Verification items for the finished model (mm, model axes). Face numbers are marked on the shaded views. A direction names the side the tool comes from. Give positions to 0.01 mm unless a question says otherwise; leave off trailing zeros. One line per question, with ' | ' between items. Start each with the question number.
Q1. Go/stop test with flat-tipped pins: pin 1 (2 mm diameter, centred on x = 43, y = -43.5, fed in from -Z); pin 2 (1 mm diameter, centred on x = 48, z = 2, fed in from -Y); pin 3 (4 mm diameter, centred on y = 26, z = 4.5, fed in from -X). Record where each tip stops, or that it passes through.
Q2. Mould release check, pull along X, two halves, no side actions. Record for the marked faces 3 and 4: released by +X, released by -X, zero draft, split by the parting line, or undercut.
Q3. Section check A-A on x = 26.5. Give the number of separate pieces and of enclosed holes in the cut face, plus the area to 3 significant figures.
Q4. Access from +Z, -Z, +X, -X, +Y, -Y to the whole of each face (thin tool, end or side, straight path). Record for the marked faces 1 and 2.
Q5. Material ranges on probe 1 along X at (y, z) = (22, 5.5); probe 2 along Y at (x, z) = (-28, 1.5); probe 3 along Y at (x, z) = (-18, 6.75), recorded low to high. Write a range as [from, to].
Autodesk Inventor part; units mm, degrees
ref_plane "Work Plane3" through (19.3185, -5.1764, 0) normal (-0.9659, 0.2588, 0) x (-0.2588, -0.9659, 0)
ref_plane "YZ Plane" through (0, 0, 0) normal (1, 0, 0) x (0, 1, 0)
ref_plane "XZ Plane" through (0, 0, 0) normal (0, 1, 0) x (-1, 0, 0)
sketch "Sketch1" plane through (0, 0, 0) normal (0, 0, 1) x (1, 0, 0)
  circle A0 centre (0, 0) radius 72.5
  circle A1 centre (0, 0) radius 67.5
  circle A2 centre (0, 0) radius 4
  line L0 (0, 20) -> (0, 60)
  arc A3 (0, 20) -> (-10, 17.3205) centre (0, 0) ccw
  line L1 (0, 0) -> (-10, 17.3205) construction
  line L2 (0, 0) -> (0, 20) construction
  arc A4 (0, 60) -> (-30, 51.9615) centre (0, 0) ccw
  line L3 (0, 0) -> (-30, 51.9615) construction
  line L4 (0, 0) -> (0, 60) construction
  line L5 (-10, 17.3205) -> (-30, 51.9615)
  line L6 (-17.3205, 10) -> (-51.9615, 30)
  arc A5 (-17.3205, 10) -> (-20, 0) centre (0, 0) ccw
  line L7 (0, 0) -> (-20, 0) construction
  line L8 (0, 0) -> (-17.3205, 10) construction
  arc A6 (-51.9615, 30) -> (-60, 0) centre (0, 0) ccw
  line L9 (0, 0) -> (-60, 0) construction
  line L10 (0, 0) -> (-51.9615, 30) construction
  line L11 (-20, 0) -> (-60, 0)
  line L12 (-17.3205, -10) -> (-51.9615, -30)
  arc A7 (-17.3205, -10) -> (-10, -17.3205) centre (0, 0) ccw
  line L13 (0, 0) -> (-10, -17.3205) construction
  line L14 (0, 0) -> (-17.3205, -10) construction
  arc A8 (-51.9615, -30) -> (-30, -51.9615) centre (0, 0) ccw
  line L15 (0, 0) -> (-30, -51.9615) construction
  line L16 (0, 0) -> (-51.9615, -30) construction
  line L17 (-10, -17.3205) -> (-30, -51.9615)
  line L18 (0, -20) -> (0, -60)
  arc A9 (0, -20) -> (10, -17.3205) centre (0, 0) ccw
  line L19 (0, 0) -> (10, -17.3205) construction
  line L20 (0, 0) -> (0, -20) construction
  arc A10 (0, -60) -> (30, -51.9615) centre (0, 0) ccw
  line L21 (0, 0) -> (30, -51.9615) construction
  line L22 (0, 0) -> (0, -60) construction
  line L23 (10, -17.3205) -> (30, -51.9615)
  line L24 (17.3205, -10) -> (51.9615, -30)
  arc A11 (17.3205, -10) -> (20, 0) centre (0, 0) ccw
  line L25 (0, 0) -> (20, 0) construction
  line L26 (0, 0) -> (17.3205, -10) construction
  arc A12 (51.9615, -30) -> (60, 0) centre (0, 0) ccw
  line L27 (0, 0) -> (60, 0) construction
  line L28 (0, 0) -> (51.9615, -30) construction
  line L29 (20, 0) -> (60, 0)
  line L30 (17.3205, 10) -> (51.9615, 30)
  arc A13 (17.3205, 10) -> (10, 17.3205) centre (0, 0) ccw
  line L31 (0, 0) -> (10, 17.3205) construction
  line L32 (0, 0) -> (17.3205, 10) construction
  arc A14 (51.9615, 30) -> (30, 51.9615) centre (0, 0) ccw
  line L33 (0, 0) -> (30, 51.9615) construction
  line L34 (0, 0) -> (51.9615, 30) construction
  line L35 (10, 17.3205) -> (30, 51.9615)
  point P0 (0, 10)
  point P1 (-2.5882, 9.6593)
  point P2 (-5, 8.6603)
  point P3 (-7.0711, 7.0711)
  point P4 (-8.6603, 5)
  point P5 (-9.6593, 2.5882)
  point P6 (-10, 0)
  point P7 (-9.6593, -2.5882)
  point P8 (-8.6603, -5)
  point P9 (-7.0711, -7.0711)
  point P10 (-5, -8.6603)
  point P11 (-2.5882, -9.6593)
  point P12 (0, -10)
  point P13 (2.5882, -9.6593)
  point P14 (5, -8.6603)
  point P15 (7.0711, -7.0711)
  point P16 (8.6603, -5)
  point P17 (9.6593, -2.5882)
  point P18 (10, 0)
  point P19 (9.6593, 2.5882)
  point P20 (8.6603, 5)
  point P21 (7.0711, 7.0711)
  point P22 (5, 8.6603)
  point P23 (2.5882, 9.6593)
  point P24 (15.5291, -57.9555)
  point P25 (30, -51.9615)
  point P26 (42.4264, -42.4264)
  point P27 (51.9615, -30)
  point P28 (57.9555, -15.5291)
  point P29 (60, 0)
  point P30 (57.9555, 15.5291)
  point P31 (51.9615, 30)
  point P32 (42.4264, 42.4264)
  point P33 (30, 51.9615)
  point P34 (15.5291, 57.9555)
  point P35 (0, 60)
  point P36 (-15.5291, 57.9555)
  point P37 (-30, 51.9615)
  point P38 (-42.4264, 42.4264)
  point P39 (-51.9615, 30)
  point P40 (-57.9555, 15.5291)
  point P41 (-60, 0)
  point P42 (-57.9555, -15.5291)
  point P43 (-51.9615, -30)
  point P44 (-42.4264, -42.4264)
  point P45 (-30, -51.9615)
  point P46 (-15.5291, -57.9555)
  dimension "d1" = 135
  dimension "d2" = 8
  dimension "d11" = 40
  dimension "d12" = 20
  dimension "d13" = 30
  dimension "d14" = 30
  dimension "d17" = 360
  dimension "d34" = 10
  dimension "d37" = 360
  dimension "d48" = 360
  dimension "d57" = 145
extrude "Extrusion1" add sketch "Sketch1" along normal blind 10 contours A1
extrude "Extrusion2" add sketch "Sketch1" along normal blind 5.5 contours A0
hole "Hole2" at (-2.5882, -9.6593, 0) at (-7.0711, 7.0711, 0) at (9.6593, 2.5882, 0) direction (0, 0, 1) diameter 4 end through all counterbore diameter 7 counterbore depth 4
hole "Hole3" at (42.4264, -42.4264, 0) at (-57.9555, -15.5291, 0) at (15.5291, 57.9555, 0) direction (0, 0, 1) diameter 4 end through all counterbore diameter 7 counterbore depth 4
chamfer "Chamfer2" distance 3.5 distance2 5 1 edges at (-72.5, 0, 5.5) measured on face at (72.06, -7.9756, 1.8333)
ref_plane "Work Plane3" through (19.3185, -5.1764, 0) normal (-0.9659, 0.2588, 0) x (-0.2588, -0.9659, 0)
sketch "Sketch3" plane through (19.3185, -5.1764, 0) normal (-0.9659, 0.2588, 0) x (-0.2588, -0.9659, 0)
  point P0 (0, 0)
  point P1 (0, 5)
  dimension "d61" = 5
hole "Hole4" at (19.3185, -5.1764, 5) direction (-0.9659, 0.2588, 0) diameter 3.5 depth 20
properties part number "wheel" material "UHMW, Black"
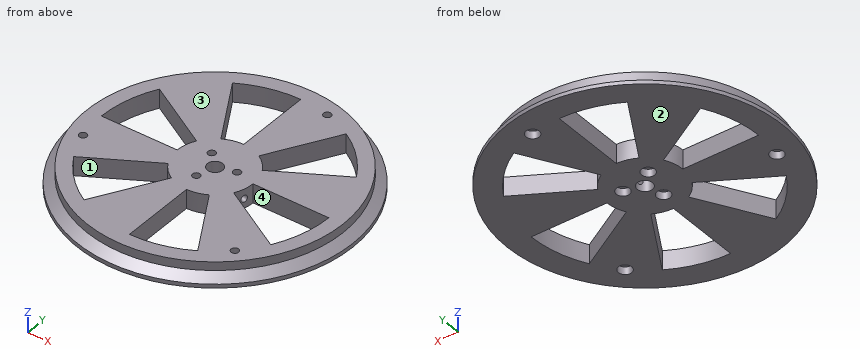
Filled in:
1) pin 1: z = 4 | pin 2: y = -54.77 | pin 3: x = -67.01
2) face 3: zero draft | face 4: undercut
3) separate pieces: 4 | enclosed holes: 0 | area: 744 mm²
4) face 1: +Z, -Z | face 2: -Z, +X, -X, +Y, -Y
5) probe 1: [-63.81, -55.82], [-38.11, -12.7], [0, 12.7], [38.11, 63.81] | probe 2: [-66.87, -48.5], [-16.17, 0], [16.17, 48.5], [53.07, 66.87] | probe 3: [-65.06, -31.18], [-10.39, 8.72], [10.39, 31.18], [57.24, 65.06]
